from build123d import *

# Parameters (mm, degrees)
F3_DEPTH = 5.08


with BuildPart() as f1:
    # F0 (on Front) → F1 (revolve)
    with BuildSketch(Plane.XZ):
        Polygon((0, 2.3735397548), (0, 0), (1.778, 0), (1.778, 2.3735397548), (10.16, 2.3735397548), (10.1363584854, 3.0589321379), (11.43, 3.103554234), (11.43, 3.4368946217), (1.778, 3.4368946217), (1.778, 5.08), (0, 5.08), (0, 3.81), (-9.906, 3.468308365), (-9.906, 3.81), (-11.176, 3.81), (-11.176, 3.175), (-4.826, 3.175), (-4.826, 2.3735397548), align=None)
    revolve(axis=Axis((0.889, 0, 0), (-1, 0, 0)))

    # F2 (on face) → F3 (cut)
    with BuildSketch(Plane(origin=(-11.176, 0, 0), x_dir=(0, -1, 0), z_dir=(-1, 0, 0))):
        with BuildLine():
            ThreePointArc((0.4744467442, 3.1393510933), (0, 3.175), (-0.4744467442, 3.1393510933))
            Line((-0.4744467442, 3.1393510933), (-0.4744467442, 1.5797834679))
            Line((-0.4744467442, 1.5797834679), (0.4744467442, 1.5797834679))
            Line((0.4744467442, 1.5797834679), (0.4744467442, 3.1393510933))
        make_face()
        with BuildLine():
            Line((0.4744467442, 4.7702165321), (-0.4744467442, 4.7702165321))
            Line((-0.4744467442, 4.7702165321), (-0.4744467442, 3.7803439376))
            ThreePointArc((-0.4744467442, 3.7803439376), (0, 3.81), (0.4744467442, 3.7803439376))
            Line((0.4744467442, 3.7803439376), (0.4744467442, 4.7702165321))
        make_face()
        with BuildLine():
            ThreePointArc((0.4744467442, 3.7803439376), (0, 3.81), (-0.4744467442, 3.7803439376))
            Line((-0.4744467442, 3.7803439376), (-0.4744467442, 3.1393510933))
            ThreePointArc((-0.4744467442, 3.1393510933), (0, 3.175), (0.4744467442, 3.1393510933))
            Line((0.4744467442, 3.1393510933), (0.4744467442, 3.7803439376))
        make_face()
    extrude(amount=-F3_DEPTH, mode=Mode.SUBTRACT)


solid = f1.part
Work out the finished part from the listing and answer in its coordinate system (mm). A direction names the side the tool comes from. Round coordinates to 2 decimals unless told otherwise and drop trailing zeros. Write each loop counter-clockwise with the first axis right and the second up, starting at its lowest first coordinate (ties: lowest second). Pieces come first, ordered by that corner, then holes. Notation, with made-up numbers: M 34.25,16.5 L 42.25,16.5 A7 ccw 42.25,27.5 Z; hole C 32.25,57.5 d5. An arc over 180 degrees is marked long. Use a Markdown table: item, result.
1) Flat-ended cylindrical pins translate along their axes: pin 1 (6 mm diameter, centred on y = 0, z = 0, fed in from +X); pin 2 (1 mm diameter, centred on x = -7.5, y = -1.5, fed in from +Z); pin 3 (0.5 mm diameter, centred on x = -7.5, z = 3.5, fed in from -Y). Find the tip coordinate at first contact, or state that the pin passes through.
Taken from the geometry:
| item | result |
|---|---|
| pin 1 | stops at x = 10.16 |
| pin 2 | stops at z = 3.41 |
| pin 3 | stops at y = -1.43 |
2) Consider line 1 (Y direction, x = 7.5, z = 0); line 2 (Y direction, x = -3.3, z = 0); line 3 (Z direction, x = -7.25, y = -2.5). Determine where each line is inside the solid, lowest interval first. Write a range as [from, to].
Taken from the geometry:
| item | result |
|---|---|
| line 1 | y = [-3.44, -2.37], [2.37, 3.44] |
| line 2 | y = [-3.7, -2.37], [2.37, 3.7] |
| line 3 | z = [-2.53, -1.96], [1.96, 2.53] |
3) The part is cut by section D-D on x = -9.5. Give the vertices of the cut face in (y, z) (3 decimals), plus the area to 3 significant figures.
Taken from the geometry:
| item | result |
|---|---|
| outline | M -0.474,3.139 L -0.474,3.45 A3.482 ccw long 0.474,3.45 L 0.474,3.139 A3.175 cw long Z |
| area | 6.13 mm2 |
4) Which of the six approach directions +Z, -Z, +X, -X, +Y, -Y give full straight-line access (tool end or side, diameter ignored) to faces 1 (the face through (0.877, 5.037, -0.661)), 2 (the face through (-5.02, -2.21, -2.89)), 3 (the face through (1.778, 0, 0)), 4 (the face through (-2.379, 0.713, 2.264)), 5 (the face through (-11.176, -3, -2))?
Taken from the geometry:
| item | result |
|---|---|
| face 1 | +X, -X |
| face 2 | none |
| face 3 | +X |
| face 4 | -X |
| face 5 | +Z, -Z, -X, +Y, -Y |
5) The part is cut by section A-A on x = 7. Give the vertices of the cut face in (y, z), plus the area to 3 significant figures.
Taken from the geometry:
| item | result |
|---|---|
| outline | C 0,0 d6.87; hole C 0,0 d4.75 |
| area | 19.4 mm2 |
6) Determine the mould class of faces 6 (the face through (-10.55, 0.161, -3.807)), 7 (the face through (0, 4, 1)), 8 (the face through (0, 0, 0)) for opening direction Y: pulls with the +Y half, pulls with the -Y half, needs draft (parallel to the pull), parting line crosses it, or undercut.
Taken from the geometry:
| item | result |
|---|---|
| face 6 | parting line crosses it |
| face 7 | needs draft |
| face 8 | undercut |
